```python
from build123d import *

# Parameters (mm, degrees)
F0_R     = 1
F1_DEPTH = 1
F2_DEPTH = 8
F3_DEPTH = 10
F4_R     = 1
F5_DEPTH = 30
F6_SIZE  = 1


with BuildPart() as f1:
    # F0 (on Top) → F1 (new body)
    with BuildSketch(Plane.XY):
        Polygon((-10, 9.5), (-10, 0), (10, 0), (10, 9.5), (10, 15), (-12, 15), (-12, 9.5), align=None)
        with Locations((-4.75, 3.5)):
            Circle(F0_R, mode=Mode.SUBTRACT)
        with Locations((4.75, 3.5)):
            Circle(F0_R, mode=Mode.SUBTRACT)
        with Locations((-4.75, 3.5)):
            Circle(F0_R)
        with Locations((4.75, 3.5)):
            Circle(F0_R)
        Polygon((-14, 0), (-10, 0), (-10, 9.5), (-12, 9.5), (-12, 15), (10, 15), (10, 9.5), (10, 0), (12, 0), (12, 17), (-14, 17), align=None)
    extrude(amount=F1_DEPTH)

    # F0 (on Top) → F2 (join)
    with BuildSketch(Plane.XY):
        Polygon((-14, 0), (-10, 0), (-10, 9.5), (-12, 9.5), (-12, 15), (10, 15), (10, 9.5), (10, 0), (12, 0), (12, 17), (-14, 17), align=None)
        with Locations((-4.75, 3.5)):
            Circle(F0_R)
        with Locations((4.75, 3.5)):
            Circle(F0_R)
    extrude(amount=F2_DEPTH)

    # F3 (cut): faces of the model
    f3_faces = [f1.faces().sort_by_distance(p)[0] for p in [
        (-4.75, 3.5, 8),
        (4.75, 3.5, 8),
    ]]
    extrude(f3_faces, amount=-F3_DEPTH, mode=Mode.SUBTRACT)

    # F4 (on face) → F5 (cut)
    with BuildSketch(Plane.YZ.offset(12)):
        with Locations((13, 4)):
            Circle(F4_R)
    extrude(amount=-F5_DEPTH, mode=Mode.SUBTRACT)

    # F6
    f6_edges = [f1.edges().sort_by_distance(p)[0] for p in [
        (-14, 17, 4),
        (12, 17, 4),
        (-14, 0, 4),
        (12, 0, 4),
    ]]
    chamfer(f6_edges, length=F6_SIZE)


solid = f1.part
```
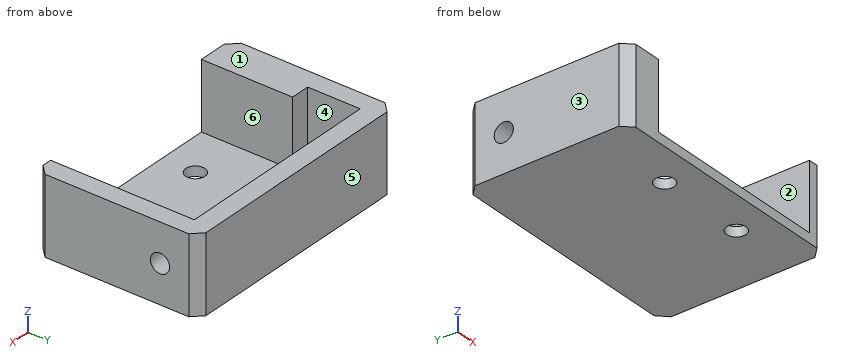
Geometry: final body of the model. Coordinates: model frame, mm. Face numbers are marked on the shaded views. A direction names the side the tool comes from. Round coordinates to 2 decimals unless told otherwise and drop trailing zeros. Write each loop counter-clockwise with the first axis right and the second up, starting at its lowest first coordinate (ties: lowest second). Pieces come first, ordered by that corner, then holes. Notation, with made-up numbers: (-13.75, -25) -> (-8.75, -25) arc R37 cw to (-8.75, 12) -> close; hole circle Ø4 at (37.25, 82.25). An arc over 180 degrees is marked (long way). Return JSON: item names as keys, results as strings.
Q1. Section D-D on y = 6.25. Return the cut outline in (x, z).
From the geometry:
{"outline": "(-14, 0) -> (12, 0) -> (12, 8) -> (10, 8) -> (10, 1) -> (-10, 1) -> (-10, 8) -> (-14, 8) -> close"}
Q2. Section A-A on y = 3.5. Return the cut outline in (x, z).
From the geometry:
{"outline": "(-14, 0) -> (-5.75, 0) -> (-5.75, 1) -> (-10, 1) -> (-10, 8) -> (-14, 8) -> close; (-3.75, 0) -> (3.75, 0) -> (3.75, 1) -> (-3.75, 1) -> close; (5.75, 0) -> (12, 0) -> (12, 8) -> (10, 8) -> (10, 1) -> (5.75, 1) -> close"}
Q3. Set-up query: the marked faces 4, 5 and 6. Return all of +Z, -Z, +X, -X, +Y, -Y with unobstructed straight access to the full face (end or side cutting, diameter ignored); none if empty.
From the geometry:
{"face 4": "+Z", "face 5": "+Z, -Z, +X, -X, +Y", "face 6": "+Z, -Y"}
Q4. Section C-C on x = 4.75. Return the cut outline in (y, z), and give its area (3 significant figures).
From the geometry:
{"outline": "(0, 0) -> (2.5, 0) -> (2.5, 1) -> (0, 1) -> close; (4.5, 0) -> (17, 0) -> (17, 8) -> (15, 8) -> (15, 1) -> (4.5, 1) -> close", "area": "29.0 mm2"}
Q5. Ray query, line 1 (X direction, y = 3.5, z = 0.45); line 2 (X direction, y = 2.25, z = 4.5); line 3 (Y direction, x = -4.75, z = 0.5). Return the intervals inside material, ascending.
From the geometry:
{"line 1": "-14 to -5.75, -3.75 to 3.75, 5.75 to 12", "line 2": "-14 to -10, 10 to 12", "line 3": "0 to 2.5, 4.5 to 17"}
Q6. Section B-B on z = 0.5. Return the cut outline in (x, y).
From the geometry:
{"outline": "(-14, 1) -> (-13, 0) -> (11, 0) -> (12, 1) -> (12, 16) -> (11, 17) -> (-13, 17) -> (-14, 16) -> close; hole circle Ø2 at (-4.75, 3.5); hole circle Ø2 at (4.75, 3.5)"}
Q7. Mould query, pull axis X, two halves, no side actions, for the marked faces 1, 2 and 3. Classes: +X half, -X half, draft (parallel to the pull), parting line (faces both ways), or undercut.
From the geometry:
{"face 1": "draft", "face 2": "undercut", "face 3": "-X half"}
Q8. First-contact query: pin 1 Ø1.2 at (y, z) = (13, 4) entering from +X; pin 2 Ø2 at (x, z) = (1, 3) entering from -Y. Flat tips, straight axial feed; report the tip coordinate or a pass-through.
From the geometry:
{"pin 1": "through", "pin 2": "y = 15"}
